CAD build for the part. Positions are in the model's coordinates, mm. Face numbers are marked on the shaded views. Round coordinates to 2 decimals unless told otherwise and drop trailing zeros. Write item = value, one per line.
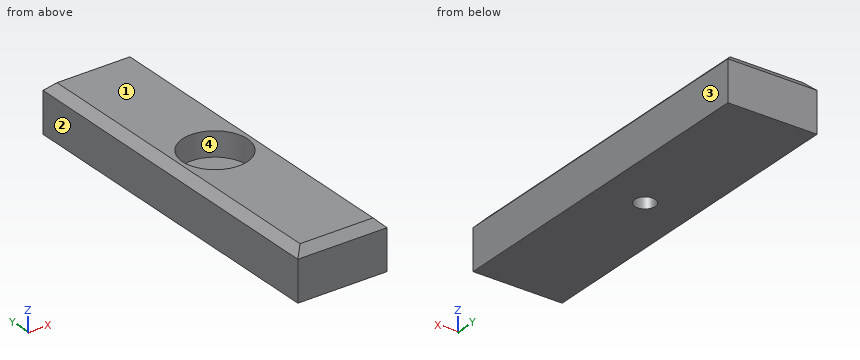
from build123d import *

# Parameters (mm, degrees)
F0_W           = 34.925
F0_H           = 136.525
F1_DEPTH       = 19.05
F2_SIZE2       = 3.175
F2_SIZE        = 3.175
F4_D           = 7.9375
F4_CBORE_D     = 25.4
F4_CBORE_DEPTH = 9.525


with BuildPart() as f1:
    # F0 (on Top) → F1 (new body)
    with BuildSketch(Plane.XY):
        Rectangle(F0_W, F0_H)
    extrude(amount=-F1_DEPTH)

    # F2
    f2_edges = [f1.edges().sort_by_distance(p)[0] for p in [
        (0, 68.2625, 0),
        (-17.4625, 0, 0),
        (0, -68.2625, 0),
        (17.4625, 0, 0),
    ]]
    chamfer(f2_edges, length=F2_SIZE, length2=F2_SIZE2)

    # F4 (through all)
    with Locations(Plane.XY):
        with Locations((0, 0)):
            CounterBoreHole(F4_D / 2, F4_CBORE_D / 2, F4_CBORE_DEPTH)


solid = f1.part
(1) Drop flat-ended pins along their axis: pin 1 (12.5 mm diameter, centred on x = 0, y = 0, fed in from +Z) (3 decimals); pin 2 (2 mm diameter, centred on y = -31, z = -2.5, fed in from +X). Give the stop position or say it passes through.
Solved:
pin_1 = -9.525
pin_2 = 17.46
(2) Probe line 1 along Y through (x, z) = (0, -14); line 2 along Y through (x, z) = (0, -6.25); line 3 along X through (y, z) = (-11, -9.25). List the from-to ranges inside material, lowest first.
Solved:
line_1 = -68.26 to -3.97, 3.97 to 68.26
line_2 = -68.26 to -12.7, 12.7 to 68.26
line_3 = -17.46 to -6.35, 6.35 to 17.46
(3) Pull direction X, two halves, no side cores. Call the marked faces 1, 2, 3 and 4: released by +X, released by -X, zero draft, split by the parting line, or undercut.
Solved:
face_1 = zero draft
face_2 = released by -X
face_3 = released by +X
face_4 = undercut
